Geometry check sheet. Reference: the model listing, model coordinates, mm. A direction names the side the tool comes from. Round coordinates to 2 decimals unless told otherwise and drop trailing zeros. Write each loop counter-clockwise with the first axis right and the second up, starting at its lowest first coordinate (ties: lowest second). Pieces come first, ordered by that corner, then holes. Notation, with made-up numbers: (72.25, 29.25) -> (115.25, 29.25) arc R24 cw to (115.25, 57.25) -> close; hole circle Ø7 at (-35.5, 61). An arc over 180 degrees is marked (long way). One line per question, with ' | ' between items.
```python
from build123d import *

# Parameters (mm, degrees)
F0_W            = 20
F0_H            = 40
F1_DEPTH        = 60
F2_R            = 5
F3_R            = 6
F4_R            = 2
F5_R            = 5.975
F6_DEPTH        = 60.001
F8_D            = 4
F8_DEPTH        = 12
F8_TIP          = 1.2017212381
F9_R            = 19
F10_DEPTH       = 25
F12_D           = 4
F12_DEPTH       = 12
F12_TIP         = 1.2017212381
F14_D           = 4
F14_DEPTH       = 12
F14_TIP         = 1.2017212381
F16_D           = 4
F16_DEPTH       = 12
F16_CSINK_D     = 10
F16_CSINK_ANGLE = 90
F16_TIP         = 1.2017212381


with BuildPart() as f1:
    # F0 (on Top) → F1 (new body)
    with BuildSketch(Plane.XY):
        Polygon((-17.5, 30.3108891325), (17.5, 30.3108891325), (31.75, 54.9926131403), (14.4294919243, 64.9926131403), (51.4294919243, 129.0784930204), (46.2333395016, 132.0784930204), (36.8527810232, 115.8308891325), (-36.8527810232, 115.8308891325), (-46.2333395016, 132.0784930204), (-51.4294919243, 129.0784930204), (-14.4294919243, 64.9926131403), (-31.75, 54.9926131403), align=None)
        with Locations((0, 56.1808891325)):
            Rectangle(F0_W, F0_H, mode=Mode.SUBTRACT)
        Polygon((34.5433799465, 111.8308891325), (18.5796450034, 84.1808891325), (-18.5796450034, 84.1808891325), (-34.5433799465, 111.8308891325), align=None, mode=Mode.SUBTRACT)
    extrude(amount=F1_DEPTH)

    # F2
    f2_edges = [f1.edges().sort_by_distance(p)[0] for p in [
        (-17.5, 30.310889, 30),
        (17.5, 30.310889, 30),
    ]]
    fillet(f2_edges, radius=F2_R)

    # F3
    f3_edges = [f1.edges().sort_by_distance(p)[0] for p in [
        (18.579645, 84.180889, 30),
        (-18.579645, 84.180889, 30),
        (-36.852781, 115.830889, 30),
        (36.852781, 115.830889, 30),
    ]]
    fillet(f3_edges, radius=F3_R)

    # F4
    f4_edges = [f1.edges().sort_by_distance(p)[0] for p in [
        (34.54338, 111.830889, 30),
        (-34.54338, 111.830889, 30),
    ]]
    fillet(f4_edges, radius=F4_R)

    # F5 (on face) → F6 (cut, through all)
    with BuildSketch(Plane.XY.offset(60)):
        with Locations((-18.8069092991, 51.5245224395)):
            Circle(F5_R)
        with Locations((18.8069092991, 51.5245224395)):
            Circle(F5_R)
    extrude(amount=-F6_DEPTH, mode=Mode.SUBTRACT)

    # F8
    with Locations(Plane(origin=(0, 115.8308891325, 0), x_dir=(-1, 0, 0), z_dir=(0, 1, 0))):
        with Locations((-23.55, 53.55), (-23.55, 6.45), (23.55, 6.45), (23.55, 53.55)):
            Hole(F8_D / 2, depth=F8_DEPTH)
            with Locations((0, 0, -(F8_DEPTH + F8_TIP / 2))):  # 118° drill point
                Cone(0, F8_D / 2, F8_TIP, mode=Mode.SUBTRACT)

    # F9 (on face) → F10 (cut)
    with BuildSketch(Plane(origin=(0, 115.8308891325, 0), x_dir=(-1, 0, 0), z_dir=(0, 1, 0))):
        with Locations((0, 30)):
            Circle(F9_R)
    extrude(amount=-F10_DEPTH, mode=Mode.SUBTRACT)

    # F12
    with Locations(Plane(origin=(-17.3205080757, 10, 0), x_dir=(0.5, 0.8660254038, 0), z_dir=(0.8660254038, -0.5, 0))):
        with Locations((92.5, 52), (129.5, 52), (92.5, 8), (129.5, 8)):
            Hole(F12_D / 2, depth=F12_DEPTH)
            with Locations((0, 0, -(F12_DEPTH + F12_TIP / 2))):  # 118° drill point
                Cone(0, F12_D / 2, F12_TIP, mode=Mode.SUBTRACT)

    # F14
    with Locations(Plane(origin=(17.3205080757, 10, 0), x_dir=(0.5, -0.8660254038, 0), z_dir=(-0.8660254038, -0.5, 0))):
        with Locations((-92.5, 8), (-129.5, 8), (-92.5, 51.9081939641), (-129.5, 51.9081939641)):
            Hole(F14_D / 2, depth=F14_DEPTH)
            with Locations((0, 0, -(F14_DEPTH + F14_TIP / 2))):  # 118° drill point
                Cone(0, F14_D / 2, F14_TIP, mode=Mode.SUBTRACT)

    # F16
    with Locations(Plane.XZ.offset(-30.3108891325)):
        with Locations((0, 10), (0, 50)):
            CounterSinkHole(F16_D / 2, F16_CSINK_D / 2, depth=F16_DEPTH, counter_sink_angle=F16_CSINK_ANGLE)
            with Locations((0, 0, -(F16_DEPTH + F16_TIP / 2))):  # 118° drill point
                Cone(0, F16_D / 2, F16_TIP, mode=Mode.SUBTRACT)


solid = f1.part
```
(1) Access from +Z, -Z, +X, -X, +Y, -Y to the whole of each face (thin tool, end or side, straight path). Record for faces 5 (the flat face through (42.463, 125.547, 29.58)), 6 (the cylindrical face through (-18.154, 85.007, 30.42)), 7 (the flat face through (-22.97, 60.06, 29.58)), 8 (the cylindrical face through (-21.642, 113.803, 7.051)).
Resolved:
face 5: +Z, -Z, +Y | face 6: +Z, -Z | face 7: +Z, -Z, -X | face 8: +Y
(2) Draft check along X on faces 1 (the flat face through (-42.356, 125.362, 29.58)), 2 (the flat face through (32.67, 96.59, 29.58)), 3 (the cylindrical face through (-17.08, 30.96, 30.42)), 4 (the cylindrical face through (-18.12, 113.86, 35.71)). Enter one of: +X half, -X half, draft (parallel to the pull), parting line (faces both ways), or undercut.
Resolved:
face 1: undercut | face 2: +X half | face 3: -X half | face 4: undercut
(3) Go/stop test with flat-tipped pins: pin 1 (4.5 mm diameter, centred on x = 0, z = 50, fed in from -Y); pin 2 (4.5 mm diameter, centred on x = 23.55, z = 6.45, fed in from -Y); pin 3 (9 mm diameter, centred on x = -3, z = 20, fed in from +Y). Record where each tip stops, or that it passes through.
Resolved:
pin 1: stops at y = 33.06 | pin 2: stops at y = 36.89 | pin 3: stops at y = 84.18
(4) Material ranges on line 1 (Z direction, x = 0, y = 34.2); line 2 (Z direction, x = 23.55, y = 114.85); line 3 (Y direction, x = 11, z = 52), recorded low to high.
Resolved:
line 1: z = 0 to 8, 12 to 48, 52 to 60 | line 2: z = 0 to 4.45, 8.45 to 51.55, 55.55 to 60 | line 3: y = 30.31 to 84.18, 111.83 to 115.83
(5) Sectioned sample at B-B on z = 30. Count the separate pieces of the cut face and the enclosed holes in it, then the cut area to 3 significant figures.
Resolved:
separate pieces: 1 | enclosed holes: 3 | area: 2,210 mm2
(6) Sectioned sample at A-A on x = 0. Record the cut outline in (y, z), then the cut area to 3 significant figures.
Resolved:
outline: (30.31, 0) -> (36.18, 0) -> (36.18, 8) -> (33.31, 8) -> (30.31, 5) -> close; (30.31, 15) -> (33.31, 12) -> (36.18, 12) -> (36.18, 48) -> (33.31, 48) -> (30.31, 45) -> close; (30.31, 55) -> (33.31, 52) -> (36.18, 52) -> (36.18, 60) -> (30.31, 60) -> close; (76.18, 0) -> (84.18, 0) -> (84.18, 60) -> (76.18, 60) -> close; (111.83, 0) -> (115.83, 0) -> (115.83, 11) -> (111.83, 11) -> close; (111.83, 49) -> (115.83, 49) -> (115.83, 60) -> (111.83, 60) -> close | area: 855 mm2
